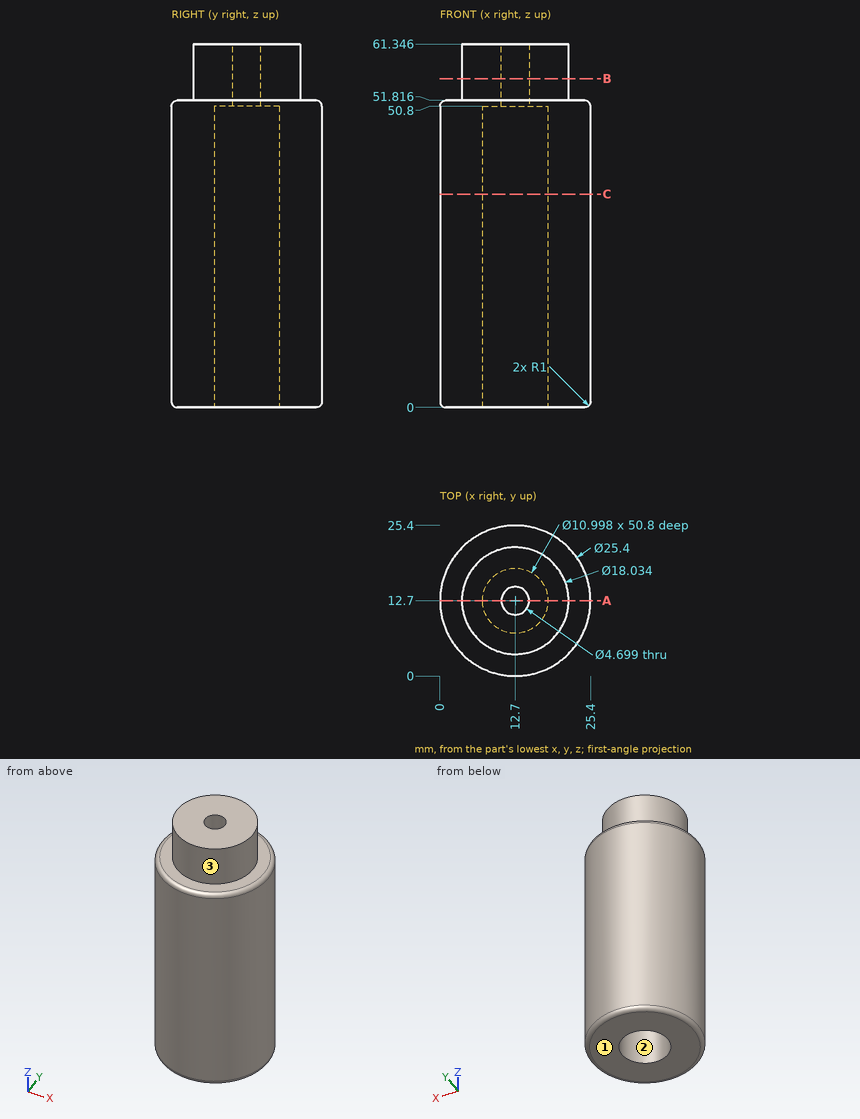
Could you check a few things on this drawing? It's one solid part, dimensions in mm from its lowest x, y, z. Coordinates: 2 decimals unless noted, no trailing zeros. Order: outer loops, then holes, each group sorted by start corner. A loop starts at its lowest first (then second) coordinate and runs counter-clockwise, first axis right, second up.
1) Imagine slicing it at C-C on z = 36. List the corners of the cut face in (x, y) for me, and give its area (3 significant figures).
2) Imagine slicing it at B-B on z = 55.5. List the corners of the cut face in (x, y) for me.
3) Imagine slicing it at A-A on y = 12.7. List the corners of the cut face in (x, z) for me.
4) I need wall thicknesses on line 1 (Y direction, x = 12.7, z = 58.5); line 2 (X direction, y = 13, z = 41.5); line 3 (Y direction, x = 12.7, z = 38.5). Which ranges of each line are inside material? Lowest first, please.
5) We'd pull the mould along X, two halves only. Please class the marked faces 1, 2 and 3: +X half, -X half, draft (parallel to the pull), parting line (faces both ways), or undercut.
6) Will these pins go through, and if not, where does the flat tip stop? pin 1 (8 mm diameter, centred on y = 18.5, z = 31, fed in from +X); pin 2 (1 mm diameter, centred on y = 3, z = 24.5, fed in from -X) (1 decimal); pin 3 (10 mm diameter, centred on x = 6.5, z = 20, fed in from -Y).
Response values:
1. outline: circle Ø25.4 at (12.7, 12.7); hole circle Ø11 at (12.7, 12.7)
1. area: 412 mm2
2. outline: circle Ø18.03 at (12.7, 12.7); hole circle Ø4.7 at (12.7, 12.7)
3. outline: (0, 1) arc R1 ccw to (1, 0) - (7.2, 0) - (7.2, 50.8) - (10.35, 50.8) - (10.35, 61.35) - (3.68, 61.35) - (3.68, 51.82) - (1, 51.82) arc R1 ccw to (0, 50.82) - close; (15.05, 50.8) - (18.2, 50.8) - (18.2, 0) - (24.4, 0) arc R1 ccw to (25.4, 1) - (25.4, 50.82) arc R1 ccw to (24.4, 51.82) - (21.72, 51.82) - (21.72, 61.35) - (15.05, 61.35) - close
4. line 1: y = 3.68 to 10.35, 15.05 to 21.72
4. line 2: x = 0 to 7.21, 18.19 to 25.4
4. line 3: y = 0 to 7.2, 18.2 to 25.4
5. face 1: draft
5. face 2: undercut
5. face 3: parting line
6. pin 1: stops at x = 25.27
6. pin 2: stops at x = 3.9
6. pin 3: stops at y = 0.06
